```python
from build123d import *

# Parameters (mm, degrees)
SKETCH1_R               = 55
BOSS_EXTRUDE1_DEPTH     = 300
CUT_EXTRUDE2_DEPTH      = 310.919344346
CUT_EXTRUDE2_DEPTH_BACK = 310.919344346
SKETCH5_R               = 50
SKETCH9_R               = 35
CUT_EXTRUDE3_DEPTH      = 211
SKETCH10_R              = 15.915907465
CUT_EXTRUDE4_DEPTH      = 177


with BuildPart() as part:
    # Sketch1 → Boss-Extrude1 (new body)
    with BuildSketch(Plane(origin=(0, 0, 0), x_dir=(1, 0, 0), z_dir=(0, 1, 0))):
        with Locations(Location((0, 0, 0), (0, 0, 270))):
            Circle(SKETCH1_R)
    extrude(amount=BOSS_EXTRUDE1_DEPTH)

    # Sketch5 → Cut-Extrude2 (cut, two sides: drawn at the far end of the back side and taken through both)
    with BuildSketch(Plane(origin=(0, 0, 0), x_dir=(0, 0, -1), z_dir=(1, 0, 0)).offset(-CUT_EXTRUDE2_DEPTH_BACK)):
        with Locations((0, 65)):
            Circle(SKETCH5_R)
    extrude(amount=CUT_EXTRUDE2_DEPTH + CUT_EXTRUDE2_DEPTH_BACK, mode=Mode.SUBTRACT)

    # Sketch9 → Cut-Extrude3 (cut)
    with BuildSketch(Plane(origin=(0, 300, 0), x_dir=(1, 0, 0), z_dir=(0, 1, 0))):
        with Locations(Location((0, 0, 0), (0, 0, 270))):
            Circle(SKETCH9_R)
    extrude(amount=-CUT_EXTRUDE3_DEPTH, mode=Mode.SUBTRACT)

    # Sketch10 → Cut-Extrude4 (cut)
    with BuildSketch(Plane.XY):
        with Locations(Location((0, 65.184966797, 0), (0, 0, 359.334121801))):
            Circle(SKETCH10_R)
    extrude(amount=-CUT_EXTRUDE4_DEPTH, mode=Mode.SUBTRACT)


solid = part.part
```
The listing builds one solid part. Answer for the finished solid, in the listing's coordinates (mm). Coordinates: 2 decimals unless noted, no trailing zeros. Loops run counter-clockwise (first coordinate to the right, second up) from the corner with the lowest first, then second, coordinate; pieces in that order, holes last. Notation, with made-up numbers: M 32,79.25 L 82,79.25 A17 ccw 82,93.25 Z; hole C 1,80.25 d4. An arc over 180 degrees is marked long. Answer as a JSON object with one key per item and string values. Group by question number.
Item 1: Consider L1, parallel to X at y = 239, z = 0; L2, parallel to X at y = 180, z = -27.5; L3, parallel to Y at x = 5.5, z = 38.5. Determine where each line is inside the solid, lowest interval first.
Item 2: Section D-D (z = 43) is taken. Write down the section's boundary in (x, y), and give its area (3 significant figures).
Item 3: Section C-C (y = 65) is taken. Write down the section's boundary in (x, z).
Item 4: Each of these flat-tipped pins is pushed along its axis until it touches: P1, Ø4, axis at x = 13.5, z = -17, coming from the +Y side; P2, Ø1, axis at y = 143, z = -26.5, coming from the +X side; P3, Ø4, axis at x = -22.5, y = 205.5, coming from the +Z side; P4, Ø3, axis at x = 43, y = 33, coming from the +Z side. Where does it stop, or does it pass through?
Item 5: Section A-A (z = 0) is taken. Write down the section's boundary in (x, y), and give its area (3 significant figures).
Item 6: Section B-B (x = -9) is taken. Write down the section's boundary in (y, z), and give its area (3 significant figures).
Item 7: Determine the mould class of faces 1 (the face through (10.513, 201.749, 33.384)), 2 (the face through (-36, 300, -1)), 3 (the face through (1, 0, -1)), 4 (the face through (14.63, 58.92, -51.11)) for opening direction Y: +Y half, -Y half, draft (parallel to the pull), parting line (faces both ways), or undercut.
Solved:
{
 "1": {"L1": "x = -55 to -35, 35 to 55", "L2": "x = -47.63 to -21.65, 21.65 to 47.63", "L3": "y = 0 to 33.1, 96.9 to 300"},
 "2": {"outline": "M -34.29,0 L 34.29,0 L 34.29,39.49 L -34.29,39.49 Z; M -34.29,90.51 L 34.29,90.51 L 34.29,300 L -34.29,300 Z", "area": "17,100 mm2"},
 "3": {"outline": "M -22.91,-50 A55 ccw -15.91,-52.65 L -15.91,-50 Z; M -22.91,50 L 22.91,50 A55 ccw Z; M 15.91,-52.65 A55 ccw 22.91,-50 L 15.91,-50 Z"},
 "4": {"P1": "stops at y = 18.75", "P2": "stops at x = 48.47", "P3": "stops at z = 51.04", "P4": "passes through"},
 "5": {"outline": "M -55,0 L 55,0 L 55,15 L -55,15 Z; M -55,115 L -35,115 L -35,300 L -55,300 Z; M 35,115 L 55,115 L 55,300 L 35,300 Z", "area": "9,050 mm2"},
 "6": {"outline": "M 0,-54.26 L 52.06,-54.26 L 52.06,-48.3 A50 cw long 101.82,33.82 L 300,33.82 L 300,54.26 L 0,54.26 Z; M 78.31,-54.26 L 300,-54.26 L 300,-33.82 L 101.82,-33.82 A50 cw 78.31,-48.2 Z", "area": "11,800 mm2"},
 "7": {"face 1": "draft", "face 2": "+Y half", "face 3": "-Y half", "face 4": "undercut"}
}
